from build123d import *


with BuildPart() as part:
    # Çizim1 → Döndür2 (revolve)
    with BuildSketch(Plane(origin=(0, 0, 0), x_dir=(0, 0, -1), z_dir=(1, 0, 0)), mode=Mode.PRIVATE) as d_nd_r2_sk:
        Polygon((-4.929577465, 10), (25.070422535, 10), (25.070422535, 15), (15.070422535, 17), (15.070422535, 24), (25.070422535, 26), (25.070422535, 30), (-4.929577465, 30), (-4.929577465, 26), (5.070422535, 24), (5.070422535, 17), (-4.929577465, 15), align=None)
    revolve(d_nd_r2_sk.sketch.rotate(Axis((0, 0, 34.929577465), (0, 0, -1)), 90), axis=Axis((0, 0, 34.929577465), (0, 0, -1)))


solid = part.part
The model under review builds one solid part; all positions refer to its coordinate system, in mm. A direction names the side the tool comes from. Coordinates: 2 decimals unless noted, no trailing zeros. Loops run counter-clockwise (first coordinate to the right, second up) from the corner with the lowest first, then second, coordinate; pieces in that order, holes last. Notation, with made-up numbers: M -39,-22 L -32,-22 A27 cw -32,12 Z; hole C 33,82 d6. An arc over 180 degrees is marked long. Put each result on its own line as item: value. Start each with the question number.
Q1. Add section C-C (z = -12). Write out the cut boundary in (x, y).
Q2. The part is to be moulded in two halves that separate along X. For faces 4 (the conical face through (-5.23, 23.551, -15.696)), 5 (the cylindrical face through (16.128, -25.296, -9.86)), 6 (the flat face through (-9, -25, 4.93)), say which applies: +X half, -X half, draft (parallel to the pull), parting line (faces both ways), or undercut.
Q3. Clearance check with flat-ended pins moving along their axes: pin 1 (12 mm diameter, centred on y = 21.5, z = -12, fed in from -X); pin 2 (1.5 mm diameter, centred on x = -9.5, z = 0.5, fed in from +Y); pin 3 (1 mm diameter, centred on x = 13.5, z = -17.5, fed in from +Y); pin 4 (18 mm diameter, centred on x = 0, y = 0, fed in from -Z). State where each tip first meets the part, or that it passes through.
Q4. For faces 1 (the flat face through (3, 10, 4.93)), 2 (the flat face through (-5.7, -16.3, -5.07)), 3 (the flat face through (5.7, -16.3, -15.07)), list the 3-axis set-ups (+Z, -Z, +X, -X, +Y, -Y) from which the entire face can be reached by the end or side of a thin tool; tool diameter is ignored.
Q5. Add section D-D (z = -20). Write out the cut boundary in (x, y).
Q6. Add section A-A (y = 0). Write out the cut boundary in (x, z), and give its area (3 significant figures).
Q7. Wall thickness on line 1 (Y direction, x = -4.5, z = -17); line 2 (Y direction, x = 0, z = -15.75); line 3 (Y direction, x = 0, z = -8): over which ranges is each line inside the solid? List them lowest first.
Answers:
1. outline: C 0,0 d60; hole C 0,0 d20
2. face 4: undercut
2. face 5: parting line
2. face 6: draft
3. pin 1: stops at x = -25.69
3. pin 2: stops at y = 28.7
3. pin 3: stops at y = 27.04
3. pin 4: passes through
4. face 1: +Z, +X, -X, +Y, -Y
4. face 2: +Z
4. face 3: -Z
5. outline: C 0,0 d60; C 0,0 d32.03; hole C 0,0 d49.97; hole C 0,0 d20
6. outline: M -30,-25.07 L -26,-25.07 L -24,-15.07 L -17,-15.07 L -15,-25.07 L -10,-25.07 L -10,4.93 L -15,4.93 L -17,-5.07 L -24,-5.07 L -26,4.93 L -30,4.93 Z; M 10,-25.07 L 15,-25.07 L 17,-15.07 L 24,-15.07 L 26,-25.07 L 30,-25.07 L 30,4.93 L 26,4.93 L 24,-5.07 L 17,-5.07 L 15,4.93 L 10,4.93 Z
6. area: 840 mm^2
7. line 1: y = -29.66 to -23.97, -15.99 to -8.93, 8.93 to 15.99, 23.97 to 29.66
7. line 2: y = -30 to -24.14, -16.86 to -10, 10 to 16.86, 24.14 to 30
7. line 3: y = -30 to -10, 10 to 30
